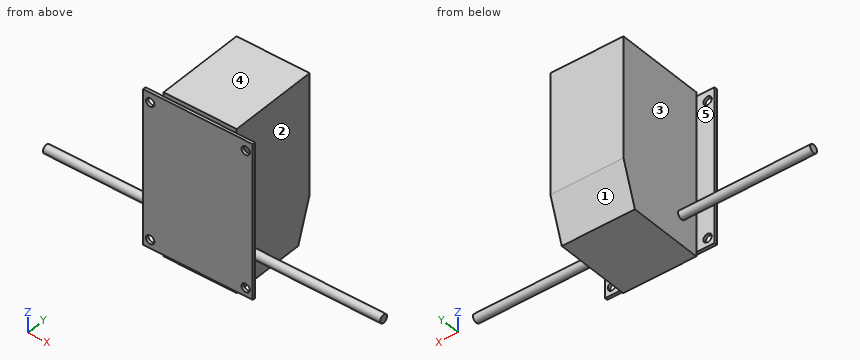
Autodesk Inventor part; units mm, degrees
ref_plane "Work Plane" through (19.5, 1, 0) normal (1, 0, 0) x (0, 0, -1)
ref_plane "YZ Plane" through (0, 0, 0) normal (1, 0, 0) x (0, 1, 0)
ref_plane "XZ Plane" through (0, 0, 0) normal (0, 1, 0) x (-1, 0, 0)
sketch "Sketch1" plane through (0, 0, 0) normal (0, 1, 0) x (-1, 0, 0)
  line L0 (0, 0) -> (-39, 0)
  line L1 (-39, 0) -> (-39, -55)
  line L2 (-39, -55) -> (0, -55)
  line L3 (0, -55) -> (0, 0)
  dimension "d228" = 39
  dimension "d229" = 55
extrude "Extrusion1" add sketch "Sketch1" along normal blind 1
sketch "Sketch2" plane through (0, 1, 0) normal (0, 1, 0) x (1, 0, 0)
  circle A0 centre (2.5, 3.5) radius 1.5
  circle A1 centre (36.5, 3.5) radius 1.5
  circle A2 centre (2.5, 52) radius 1.5
  circle A3 centre (36.5, 52) radius 1.5
  line L0 (0, 55) -> (0, 0)
  line L1 (39, 55) -> (0, 55)
  line L2 (39, 0) -> (39, 55)
  dimension "d232" = 3
  dimension "d236" = 3.5
  dimension "d237" = 2.5
  dimension "d238" = 3
  dimension "d239" = 2.5
hole "Hole1" at (2.5, 1, -3.5) at (2.5, 1, -52) at (36.5, 1, -52) at (36.5, 1, -3.5) direction (0, -1, 0) diameter 3 end through all
sketch "Sketch3" plane through (0, 1, 0) normal (0, 1, 0) x (1, 0, 0)
  line L0 (0, 0) -> (39, 0)
  line L1 (39, 55) -> (0, 55)
  line L2 (6.5, 56.5) -> (32.5, 56.5)
  line L3 (32.5, 56.5) -> (32.5, -1.5)
  line L4 (32.5, -1.5) -> (6.5, -1.5)
  line L5 (6.5, -1.5) -> (6.5, 56.5)
  dimension "d257" = 26
  dimension "d258" = 58
  dimension "d259" = 6.5
  dimension "d260" = 1.5
extrude "Extrusion2" add sketch "Sketch3" along normal blind 32
chamfer "Chamfer1" distance 15 distance2 5 1 edges at (19.5, 33, -56.5) measured on face at (15.1667, 33, -37.1667)
ref_plane "Work Plane" through (19.5, 1, 0) normal (1, 0, 0) x (0, 0, -1)
sketch "Sketch4" plane through (19.5, 1, 0) normal (1, 0, 0) x (0, 0, -1)
  circle A0 centre (46, 6.5) radius 1.5
  line L0 (56.5, 0) -> (56.5, 27)
  line L1 (0, 0) -> (55, 0)
  point P0 (0, -1)
  dimension "d272" = 3
  dimension "d273" = 10.5
  dimension "d274" = 6.5
extrude "Extrusion3" add sketch "Sketch4" along normal mid plane 120
properties part number "Langbektang houder"
Verification items for the finished model (mm, model axes). Face numbers are marked on the shaded views. A direction names the side the tool comes from. Give positions to 0.01 mm unless a question says otherwise; leave off trailing zeros. Loops run counter-clockwise (first coordinate to the right, second up) from the corner with the lowest first, then second, coordinate; pieces in that order, holes last.
1) Thickness scan on line 1 along X through (y, z) = (0.55, -3.5); line 2 along Z through (x, y) = (2.5, 0.45); line 3 along X through (y, z) = (23.5, -22). Record the ranges inside material, lowest first.
2) Depth check by flat-ended pin: pin 1 Ø3 at (x, z) = (36, -30.5) entering from +Y; pin 2 Ø8 at (x, y) = (-15, 12) entering from +Z; pin 3 Ø4 at (x, y) = (44, 6) entering from +Z. Enter the tip coordinate at first touch or a pass-through.
3) Sectioned sample at B-B, the plane x = 36.5. Enter the section's corners in (y, z).
4) Sectioned sample at C-C, the plane z = -46. Enter the section's corners in (x, y), then the cut area to 3 significant figures.
5) Sectioned sample at D-D, the plane y = 7.5. Enter the section's corners in (x, z), then the cut area to 3 significant figures.
6) Draft check along X on the marked faces 1, 2 and 3. Enter one of: pulls with the +X half, pulls with the -X half, needs draft (parallel to the pull), parting line crosses it, or undercut.
7) Sectioned sample at A-A, the plane z = -3.5. Enter the section's corners in (x, y).
8) Set-up check for the marked faces 4 and 5: record each of +Z, -Z, +X, -X, +Y, -Y from which the full face is reachable in a straight line by a thin tool's end or side.
Answers:
1. line 1: x = 0 to 1, 4 to 35, 38 to 39
1. line 2: z = -55 to -53.5, -50.5 to -5, -2 to 0
1. line 3: x = 6.5 to 32.5
2. pin 1: stops at y = 1
2. pin 2: stops at z = -44.59
2. pin 3: stops at z = -44.5
3. outline: (0, -55) - (1, -55) - (1, -53.5) - (0, -53.5) - close; (0, -50.5) - (1, -50.5) - (1, -5) - (0, -5) - close; (0, -2) - (1, -2) - (1, 0) - (0, 0) - close; circle Ø3 at (7.5, -46)
4. outline: (-40.5, 6) - (6.5, 6) - (6.5, 1) - (0, 1) - (0, 0) - (39, 0) - (39, 1) - (32.5, 1) - (32.5, 6) - (79.5, 6) - (79.5, 9) - (32.5, 9) - (32.5, 31.5) - (6.5, 31.5) - (6.5, 9) - (-40.5, 9) - close
4. area: 1,110 mm2
5. outline: (-40.5, -47.5) - (6.5, -47.5) - (6.5, -56.5) - (32.5, -56.5) - (32.5, -47.5) - (79.5, -47.5) - (79.5, -44.5) - (32.5, -44.5) - (32.5, 1.5) - (6.5, 1.5) - (6.5, -44.5) - (-40.5, -44.5) - close
5. area: 1,790 mm2
6. face 1: needs draft
6. face 2: pulls with the +X half
6. face 3: pulls with the -X half
7. outline: (0, 0) - (1, 0) - (1, 1) - (0, 1) - close; (4, 0) - (35, 0) - (35, 1) - (32.5, 1) - (32.5, 33) - (6.5, 33) - (6.5, 1) - (4, 1) - close; (38, 0) - (39, 0) - (39, 1) - (38, 1) - close
8. face 4: +Z, +X, -X, +Y, -Y
8. face 5: +Z, -Z, -X
